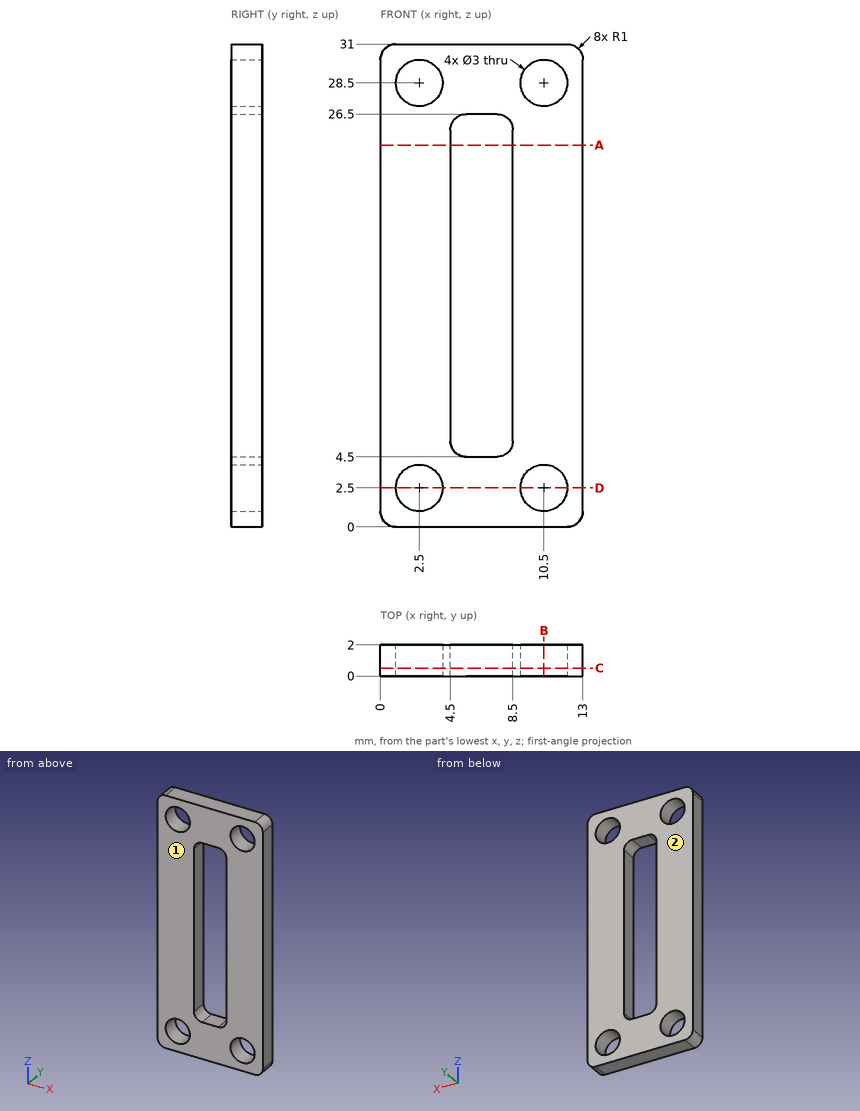
Drawing for the job (mm, zero at the part's lowest x, y, z). Give positions to 0.01 mm unless a question says otherwise; leave off trailing zeros. Loops run counter-clockwise (first coordinate to the right, second up) from the corner with the lowest first, then second, coordinate; pieces in that order, holes last. Notation, with made-up numbers: (56.5, 59.25) - (109.5, 59.25) arc R19 cw to (109.5, 69.25) - close; hole circle Ø4 at (28.5, 18). An arc over 180 degrees is marked (long way). Write item = value, one per line. Start each with the question number.
1) Pull direction Y, two halves, no side cores. Call the marked faces 1 and 2: +Y half, -Y half, draft (parallel to the pull), parting line (faces both ways), or undercut.
2) Probe probe 1 along Z at (x, y) = (2.5, 1.2); probe 2 along X at (y, z) = (1.1, 28.5); probe 3 along X at (y, z) = (0.7, 20). List the from-to ranges inside material, lowest first. Write a range as from..to.
3) Band-saw the part on C-C on y = 0.5. Give the cut face in (x, z).
4) Band-saw the part on A-A on z = 24.5. Give the cut face in (x, y), plus the area to 3 significant figures.
5) Band-saw the part on D-D on z = 2.5. Give the cut face in (x, y), plus the area to 3 significant figures.
6) Band-saw the part on B-B on x = 10.5. Give the cut face in (y, z).
Final values:
q1.face_1 = -Y half
q1.face_2 = +Y half
q2.probe_1 = 0..1, 4..27, 30..31
q2.probe_2 = 0..1, 4..9, 12..13
q2.probe_3 = 0..4.5, 8.5..13
q3.outline = (0, 1) arc R1 ccw to (1, 0) - (12, 0) arc R1 ccw to (13, 1) - (13, 30) arc R1 ccw to (12, 31) - (1, 31) arc R1 ccw to (0, 30) - close; hole circle Ø3 at (2.5, 2.5); hole circle Ø3 at (2.5, 28.5); hole (4.5, 5.5) arc R1 ccw to (5.5, 4.5) - (7.5, 4.5) arc R1 ccw to (8.5, 5.5) - (8.5, 25.5) arc R1 ccw to (7.5, 26.5) - (5.5, 26.5) arc R1 ccw to (4.5, 25.5) - close; hole circle Ø3 at (10.5, 2.5); hole circle Ø3 at (10.5, 28.5)
q4.outline = (0, 0) - (4.5, 0) - (4.5, 2) - (0, 2) - close; (8.5, 0) - (13, 0) - (13, 2) - (8.5, 2) - close
q4.area = 18.0 mm²
q5.outline = (0, 0) - (1, 0) - (1, 2) - (0, 2) - close; (4, 0) - (9, 0) - (9, 2) - (4, 2) - close; (12, 0) - (13, 0) - (13, 2) - (12, 2) - close
q5.area = 14.0 mm²
q6.outline = (0, 0) - (2, 0) - (2, 1) - (0, 1) - close; (0, 4) - (2, 4) - (2, 27) - (0, 27) - close; (0, 30) - (2, 30) - (2, 31) - (0, 31) - close
